Build history of the part. All positions in model axes, mm. Face numbers are marked on the shaded views. A direction names the side the tool comes from. Round coordinates to 2 decimals unless told otherwise and drop trailing zeros. Write each loop counter-clockwise with the first axis right and the second up, starting at its lowest first coordinate (ties: lowest second). Pieces come first, ordered by that corner, then holes. Notation, with made-up numbers: (9.5, 42) - (21.5, 42) arc R25 cw to (21.5, 59) - close; hole circle Ø2 at (75.25, 9.25). An arc over 180 degrees is marked (long way). Answer as a JSON object with one key per item and string values. Group by question number.
Item 1: Slice it at A-A, the plane x = 0. List the corners of the cut face in (y, z), then the cut area to 4 significant figures.
Item 2: Slice it at C-C, the plane z = 7. List the corners of the cut face in (x, y), then the cut area to 3 significant figures.
Item 3: Two-plate mould, pull along X, no slides. Class the marked faces 4, 5 and 6: +X half, -X half, draft (parallel to the pull), parting line (faces both ways), or undercut.
Item 4: Probe line 1 (Y direction, x = -10.5, z = 3.75); line 2 (X direction, y = -8.5, z = 1.75); line 3 (X direction, y = 5, z = 1). List the from-to ranges inside material, lowest first. Write a range as from..to.
Item 5: Which spindle directions (+Z, -Z, +X, -X, +Y, -Y) get a long thin tool onto all of the face, cutting with end or side? Do the marked faces 1, 2 and 3. Say none if no direction does.
Item 6: Slice it at B-B, the plane z = 1.5. List the corners of the cut face in (x, y), then the cut area to 3 significant figures.
Item 7: Flat gauge pins, fed straight in: pin 1 (1 mm diameter, centred on x = 2, z = 7, fed in from -Y); pin 2 (19 mm diameter, centred on x = 0, y = 0, fed in from -Z) (3 decimals); pin 3 (6.5 mm diameter, centred on x = -12, y = -12.5, fed in from -Z); pin 4 (3.5 mm diameter, centred on x = 11.85, y = 11.85, fed in from +Z). Where does each tip first touch, or does it go through?
from build123d import *

# Parameters (mm, degrees)
SKETCH1_R           = 1.5
SKETCH1_R_2         = 12
BOSS_EXTRUDE1_DEPTH = 9
SKETCH2_R           = 14
CUT_EXTRUDE1_DEPTH  = 4
SKETCH3_R           = 4
CUT_EXTRUDE2_DEPTH  = 3
CHAMFER1_SIZE       = 0.5
CHAMFER2_SIZE       = 0.5


with BuildPart() as part:
    # Sketch1 → Boss-Extrude1 (new body)
    with BuildSketch(Plane.XY):
        with BuildLine():
            Line((-14.5, 17), (14.5, 17))
            ThreePointArc((14.5, 17), (15.799525309, 15.799525309), (17, 14.5))
            Line((17, 14.5), (17, -14.5))
            ThreePointArc((17, -14.5), (15.799525309, -15.799525309), (14.5, -17))
            Line((14.5, -17), (-14.5, -17))
            ThreePointArc((-14.5, -17), (-15.799525309, -15.799525309), (-17, -14.5))
            Line((-17, -14.5), (-17, 14.5))
            ThreePointArc((-17, 14.5), (-15.799525309, 15.799525309), (-14.5, 17))
        make_face()
        with Locations((-11.85, 11.85)):
            Circle(SKETCH1_R, mode=Mode.SUBTRACT)
        with Locations((11.85, 11.85)):
            Circle(SKETCH1_R, mode=Mode.SUBTRACT)
        with Locations((11.85, -11.85)):
            Circle(SKETCH1_R, mode=Mode.SUBTRACT)
        with Locations((-11.85, -11.85)):
            Circle(SKETCH1_R, mode=Mode.SUBTRACT)
        Circle(SKETCH1_R_2, mode=Mode.SUBTRACT)
    extrude(amount=BOSS_EXTRUDE1_DEPTH)

    # Sketch2 → Cut-Extrude1 (cut)
    with BuildSketch(Plane.XY.offset(9)):
        with BuildLine():
            Line((-14.5, 17), (14.5, 17))
            ThreePointArc((14.5, 17), (15.799525309, 15.799525309), (17, 14.5))
            Line((17, 14.5), (17, -14.5))
            ThreePointArc((17, -14.5), (15.799525309, -15.799525309), (14.5, -17))
            Line((14.5, -17), (-14.5, -17))
            ThreePointArc((-14.5, -17), (-15.799525309, -15.799525309), (-17, -14.5))
            Line((-17, -14.5), (-17, 14.5))
            ThreePointArc((-17, 14.5), (-15.799525309, 15.799525309), (-14.5, 17))
        make_face()
        Circle(SKETCH2_R, mode=Mode.SUBTRACT)
    extrude(amount=-CUT_EXTRUDE1_DEPTH, mode=Mode.SUBTRACT)

    # Sketch3 → Cut-Extrude2 (cut)
    with BuildSketch(Plane(origin=(0, 0, 0), x_dir=(-1, 0, 0), z_dir=(0, 0, -1))):
        with Locations((-11.85, 11.85)):
            Circle(SKETCH3_R)
        with Locations((11.85, 11.85)):
            Circle(SKETCH3_R)
        with Locations((11.85, -11.85)):
            Circle(SKETCH3_R)
        with Locations((-11.85, -11.85)):
            Circle(SKETCH3_R)
    extrude(amount=-CUT_EXTRUDE2_DEPTH, mode=Mode.SUBTRACT)

    # Chamfer1
    chamfer1_edges = [part.edges().sort_by_distance(p)[0] for p in [
        (-17, 0, 0),
        (-15.799525309, 15.799525309, 0),
        (-15.799525309, 15.799525309, 5),
        (0, 17, 5),
        (15.799525309, 15.799525309, 5),
        (17, 0, 5),
        (15.799525309, -15.799525309, 5),
        (0, -17, 5),
        (-15.799525309, -15.799525309, 5),
        (-17, 0, 5),
        (0, 17, 0),
        (15.799525309, 15.799525309, 0),
        (17, 0, 0),
        (15.799525309, -15.799525309, 0),
        (0, -17, 0),
        (-15.799525309, -15.799525309, 0),
    ]]
    chamfer(chamfer1_edges, length=CHAMFER1_SIZE)

    # Chamfer2
    chamfer2_edges = [part.edges().sort_by_distance(p)[0] for p in [
        (-12, 0, 0),
        (-12, 0, 9),
        (-14, 0, 9),
    ]]
    chamfer(chamfer2_edges, length=CHAMFER2_SIZE)


solid = part.part
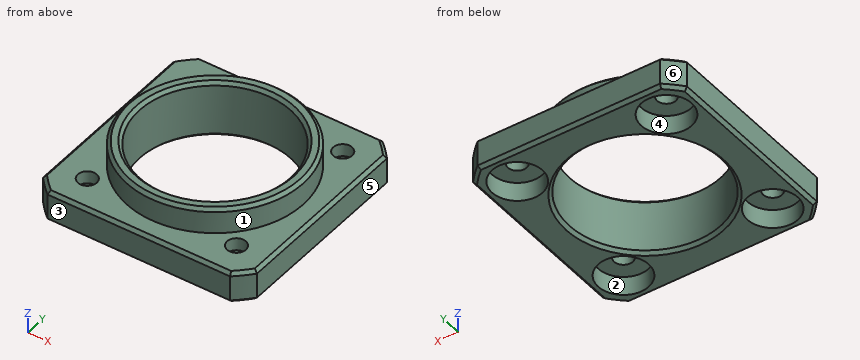
Geometry says:
{
 "1": {"outline": "(-17, 0.5) - (-16.5, 0) - (-12.5, 0) - (-12, 0.5) - (-12, 8.5) - (-12.5, 9) - (-13.5, 9) - (-14, 8.5) - (-14, 5) - (-16.5, 5) - (-17, 4.5) - close; (12, 0.5) - (12.5, 0) - (16.5, 0) - (17, 0.5) - (17, 4.5) - (16.5, 5) - (14, 5) - (14, 8.5) - (13.5, 9) - (12.5, 9) - (12, 8.5) - close", "area": "64.75 mm^2"},
 "2": {"outline": "circle Ø28 at (0, 0); hole circle Ø24 at (0, 0)", "area": "163 mm^2"},
 "3": {"face 4": "undercut", "face 5": "+X half", "face 6": "-X half"},
 "4": {"line 1": "y = -17..-12.5, -11.2..-5.81, 5.81..11.2, 12.5..17", "line 2": "x = -17..-14.04, -9.66..-8.47, 8.47..9.66, 14.04..17", "line 3": "x = -17..-10.91, 10.91..17"},
 "5": {"face 1": "+Z", "face 2": "-Z", "face 3": "+Z, -Z, +X, -X, -Y"},
 "6": {"outline": "(-17, -14.5) arc R22.34 ccw to (-14.5, -17) - (14.5, -17) arc R22.34 ccw to (17, -14.5) - (17, 14.5) arc R22.34 ccw to (14.5, 17) - (-14.5, 17) arc R22.34 ccw to (-17, 14.5) - close; hole circle Ø8 at (-11.85, -11.85); hole circle Ø8 at (-11.85, 11.85); hole circle Ø24 at (0, 0); hole circle Ø8 at (11.85, -11.85); hole circle Ø8 at (11.85, 11.85)", "area": "491 mm^2"},
 "7": {"pin 1": "stops at y = -13.92", "pin 2": "passes through", "pin 3": "stops at z = 3", "pin 4": "stops at z = 5"}
}
